Design review of the part built by this model. Coordinates are the model's own, in mm. A direction names the side the tool comes from. Give positions to 0.01 mm unless a question says otherwise; leave off trailing zeros. Loops run counter-clockwise (first coordinate to the right, second up) from the corner with the lowest first, then second, coordinate; pieces in that order, holes last.
from build123d import *

# Parameters (mm, degrees)
BOSS_EXTRUDE1_DEPTH  = 27.5
BOSS_EXTRUDE2_DEPTH  = 4.2545
LPATTERN2_COUNT      = 2
LPATTERN2_PITCH      = 65.405
MIRROR2_COPY_1_DEPTH = 4.2545


with BuildPart() as part:
    # Sketch1 → Boss-Extrude1 (new body)
    with BuildSketch(Plane.XY):
        with BuildLine():
            Line((0, 0), (-79.276260795, 0))
            ThreePointArc((-79.276260795, 0), (-79.053846694, 0.797858902), (-78.803819102, 1.5875))
            Line((-78.803819102, 1.5875), (-0.472441693, 1.5875))
            ThreePointArc((-0.472441693, 1.5875), (-0.222414101, 0.797858902), (0, 0))
        make_face()
    extrude(amount=BOSS_EXTRUDE1_DEPTH)

    # 3DSketch1 → Boss-Extrude2 (add)
    with BuildSketch(Plane(origin=(-4.808380397, 1.5875, 27.5), x_dir=(0, 0.9555235878955425, -0.2949146876220808), z_dir=(1, 0, 0))):
        Polygon((0, 0), (2.487705661, 0.767810389), (2.019528594, 2.284704085), (5.148824108, 0.758446848), (5.382912641, 0), (0.468177067, -1.516893696), align=None)
    boss_extrude2 = extrude(amount=-BOSS_EXTRUDE2_DEPTH)

    # LPattern2: Boss-Extrude2 ×2
    with Locations(*[(-i * LPATTERN2_PITCH, 0, 0) for i in range(1, LPATTERN2_COUNT)]):
        add(boss_extrude2)

    # Mirror2: Boss-Extrude2 across plane
    add(boss_extrude2.mirror(Plane.XY.offset(13.750000068)))

    # Mirror2 copy 1 sketch → Mirror2 copy 1 (add)
    with BuildSketch(Plane(origin=(-70.213380397, 1.5875, 1.36e-07), x_dir=(0, 0.9555235878955425, 0.2949146876220808), z_dir=(1, 0, 0))):
        Polygon((0, 0), (2.487705661, -0.767810389), (2.019528594, -2.284704085), (5.148824108, -0.758446848), (5.382912641, 0), (0.468177067, 1.516893696), align=None)
    extrude(amount=-MIRROR2_COPY_1_DEPTH)


solid = part.part
Q1. Insertion check: pin 1 (1.3 mm diameter, centred on x = -27.5, y = 1, fed in from -Z); pin 2 (2.5 mm diameter, centred on y = 4.5, z = 27, fed in from -X); pin 3 (3.5 mm diameter, centred on y = 4, z = 27.5, fed in from +X). Each pin has a flat end and moves straight along its axis. Give the tip position at first contact, or say it passes through.
Results:
pin 1: stops at z = 0
pin 2: stops at x = -74.47
pin 3: stops at x = -4.81
Q2. Draft analysis for pull direction X (two halves, no side actions). For faces 6 (the face through (-70.213, 4.2, 0.4)), 7 (the face through (-0.226, 0.809, 13.558)), 8 (the face through (-72, 4, 1.588)), 9 (the face through (-9.063, 4, 27)), state which applies: pulls with the +X half, pulls with the -X half, needs draft (parallel to the pull), parting line crosses it, or undercut.
Results:
face 6: undercut
face 7: pulls with the +X half
face 8: needs draft
face 9: undercut
Q3. Take a section at C-C (z = 20). Give the boundary of the cut face in (x, y) (1 decimal), plus the area to 3 significant figures.
Results:
outline: (-79.3, 0) - (0, 0) arc R23.8 ccw to (-0.5, 1.6) - (-78.8, 1.6) arc R23.8 ccw to start
area: 125 mm2
Q4. Take a section at B-B (x = -6.5). Give the boundary of the cut face in (y, z), plus the area to 3 significant figures.
Results:
outline: (0, 0) - (4.19, 0) - (4.19, -1.59) - (6.73, 0.79) - (6.73, 1.59) - (1.59, 1.59) - (1.59, 25.91) - (6.73, 25.91) - (6.73, 26.71) - (4.19, 29.09) - (4.19, 27.5) - (0, 27.5) - close
area: 62.0 mm2
Q5. Tool access review of faces 1 (the face through (-72, 4.191, -1)), 2 (the face through (-7, 4.191, 28)), 3 (the face through (-4.808, 4, 1)), 4 (the face through (-72, 4, 25.912)), 5 (the face through (-70.213, 4, 27)): name each direction out of +Z, -Z, +X, -X, +Y, -Y from which nothing blocks a thin tool from reaching the whole face with its end or side.
Results:
face 1: -Z, +X, -X, -Y
face 2: +Z, +X, -X, -Y
face 3: +Z, -Z, +X, +Y
face 4: +X, -X, +Y
face 5: +Z, -Z, +Y
Q6. Take a section at D-D (y = 6). Give the boundary of the cut face in (x, z).
Results:
outline: (-74.47, 0.11) - (-70.21, 0.11) - (-70.21, 1.59) - (-74.47, 1.59) - close; (-74.47, 25.91) - (-70.21, 25.91) - (-70.21, 27.39) - (-74.47, 27.39) - close; (-9.06, 0.11) - (-4.81, 0.11) - (-4.81, 1.59) - (-9.06, 1.59) - close; (-9.06, 25.91) - (-4.81, 25.91) - (-4.81, 27.39) - (-9.06, 27.39) - close
Q7. Take a section at A-A (y = 2.75). Give the boundary of the cut face in (x, z).
Results:
outline: (-74.47, 0) - (-70.21, 0) - (-70.21, 1.59) - (-74.47, 1.59) - close; (-74.47, 25.91) - (-70.21, 25.91) - (-70.21, 27.5) - (-74.47, 27.5) - close; (-9.06, 0) - (-4.81, 0) - (-4.81, 1.59) - (-9.06, 1.59) - close; (-9.06, 25.91) - (-4.81, 25.91) - (-4.81, 27.5) - (-9.06, 27.5) - close
Q8. Wall thickness on line 1 (X direction, y = 4.75, z = 26); line 2 (Y direction, x = -66.5, z = 20.5); line 3 (Z direction, x = -49, y = 0.5): over which ranges is each line inside the solid? List them lowest first.
Results:
line 1: x = -74.47 to -70.21, -9.06 to -4.81
line 2: y = 0 to 1.59
line 3: z = 0 to 27.5
